Design review of the part built by this model. Coordinates are the model's own, in mm. A direction names the side the tool comes from. Give positions to 0.01 mm unless a question says otherwise; leave off trailing zeros. Write each loop counter-clockwise with the first axis right and the second up, starting at its lowest first coordinate (ties: lowest second). Pieces come first, ordered by that corner, then holes.
```python
from build123d import *

# Parameters (mm, degrees)
SALIENTE_EXTRUIR1_DEPTH = 1.25
CHAFL_N1_SIZE           = 1.5
CHAFL_N2_SIZE           = 6
CHAFL_N2_SIZE2          = 3
REDONDEO1_R             = 2
REDONDEO2_R             = 10
REDONDEO2_2_R           = 5
REDONDEO3_R             = 0.8
CROQUIS6_R              = 1.2
CROQUIS6_R_2            = 1.7
CORTAR_EXTRUIR1_DEPTH   = 3.5


with BuildPart() as part:
    # Croquis5 → Saliente-Extruir1 (new body, symmetric)
    with BuildSketch(Plane.XY):
        Polygon((-33.3960961, -67.058199354), (-49.468312924, -54.332876319), (-49.042492677, -42.832876319), (-75.361903804, -2.692016862), (-89.503725327, 7.973817187), (-89.503725327, 13.973817187), (-83.503725327, 13.973817187), (-83.503725327, 33.973817187), (-108.003725327, 33.973817187), (-113.503725327, 33.973817187), (-113.503725327, 40.973817187), (-83.503725327, 40.973817187), (-76.07625416, 40.973817187), (-46.8531225, 19.949817187), (-27.852472036, -53.120185426), (-23.157930014, -60.798809991), align=None)
        Polygon((-51.475681089, 9.911759166), (-40.150790084, -33.639898021), (-44.730652374, -36.642805286), (-66.937655512, -2.77395512), align=None, mode=Mode.SUBTRACT)
        Polygon((-72.503725327, 4.947596176), (-56.268652183, 18.267596176), (-72.503725327, 29.947596176), align=None, mode=Mode.SUBTRACT)
    extrude(amount=SALIENTE_EXTRUIR1_DEPTH, both=True)

    # Chafl_n1
    chafl_n1_edges = [part.edges().sort_by_distance(p)[0] for p in [
        (-113.503725327, 33.973817187, 0),
        (-89.503725327, 13.973817187, 0),
    ]]
    chamfer(chafl_n1_edges, length=CHAFL_N1_SIZE)

    # Chafl_n2
    chafl_n2_edges = [part.edges().sort_by_distance(p)[0] for p in [
        (-113.503725327, 40.973817187, 0),
    ]]
    chafl_n2_side = [part.faces().sort_by_distance(p)[0] for p in [
        (-94.789989743, 40.973817187, 0),
    ]]
    chamfer(chafl_n2_edges, length=CHAFL_N2_SIZE, length2=CHAFL_N2_SIZE2, reference=chafl_n2_side[0])

    # Redondeo1
    redondeo1_edges = [part.edges().sort_by_distance(p)[0] for p in [
        (-23.157930014, -60.798809991, 0),
        (-33.3960961, -67.058199354, 0),
        (-51.475681089, 9.911759166, 0),
        (-66.937655512, -2.77395512, 0),
        (-44.730652374, -36.642805286, 0),
        (-40.150790084, -33.639898021, 0),
        (-56.268652183, 18.267596176, 0),
        (-72.503725327, 29.947596176, 0),
        (-72.503725327, 4.947596176, 0),
    ]]
    fillet(redondeo1_edges, radius=REDONDEO1_R)

    # Redondeo2
    redondeo2_edges = [part.edges().sort_by_distance(p)[0] for p in [
        (-76.07625416, 40.973817187, 0),
        (-46.8531225, 19.949817187, 0),
        (-75.361903804, -2.692016862, 0),
        (-27.852472036, -53.120185426, 0),
        (-49.042492677, -42.832876319, 0),
    ]]
    fillet(redondeo2_edges, radius=REDONDEO2_R)

    # Redondeo2 2
    redondeo2_2_edges = [part.edges().sort_by_distance(p)[0] for p in [
        (-49.468312924, -54.332876319, 0),
    ]]
    fillet(redondeo2_2_edges, radius=REDONDEO2_2_R)

    # Redondeo3
    redondeo3_edges = [part.edges().sort_by_distance(p)[0] for p in [
        (-83.503725327, 13.973817187, 0),
        (-83.503725327, 33.973817187, 0),
    ]]
    fillet(redondeo3_edges, radius=REDONDEO3_R)

    # Croquis6 → Cortar-Extruir1 (cut, through all)
    with BuildSketch(Plane.XY.offset(1.25)):
        with Locations((-80.003725327, 31.973817187)):
            Circle(CROQUIS6_R)
        with Locations((-80.003725327, 15.973817187)):
            Circle(CROQUIS6_R)
        with Locations((-85.503725327, 37.473817187)):
            Circle(CROQUIS6_R)
        with Locations((-93.503725327, 37.473817187)):
            Circle(CROQUIS6_R)
        with Locations((-101.503725327, 37.473817187)):
            Circle(CROQUIS6_R)
        with Locations((-109.503725327, 37.473817187)):
            Circle(CROQUIS6_R)
        with Locations((-85.503725327, 10.473817187)):
            Circle(CROQUIS6_R)
        with Locations((-51.75750024, 15.82464715)):
            Circle(CROQUIS6_R_2)
        with Locations((-36.753725327, -37.919792915)):
            Circle(CROQUIS6_R_2)
        with Locations((-44.377518673, -51.986696449)):
            Circle(CROQUIS6_R_2)
        Polygon((-39.612609009, -53.277564811), (-33.640345459, -49.626254349), (-38.856503262, -41.094449277), (-44.828766812, -44.745759739), align=None)
    extrude(amount=-CORTAR_EXTRUIR1_DEPTH, mode=Mode.SUBTRACT)


solid = part.part
```
(1) To check wall thickness, follow L1, parallel to Y at x = -93.5, z = 0; L2, parallel to Y at x = -59, z = -1; L3, parallel to Y at x = -59.5, z = 0.35. State the ranges of each line that lie inside material, in increasing order.
Resolved:
L1: y = 33.97 to 36.27, 38.67 to 40.97
L2: y = -27.65 to -14.88, 3.74 to 16.03, 20.23 to 28.69
L3: y = -26.88 to -14.12, 3.33 to 15.62, 20.59 to 29.05
(2) Clearance check with flat-ended pins moving along their axes: P1, Ø2, axis at x = -101.5, y = 37.47, coming from the +Z side; P2, Ø6, axis at x = -35.5, y = -21, coming from the +Z side; P3, Ø1.5, axis at y = -28, z = -0.5, coming from the +X side; P4, Ø1.5, axis at y = -39, z = -1, coming from the -X side. State where each tip first meets the part, or that it passes through.
Resolved:
P1: passes through
P2: stops at z = 1.25
P3: stops at x = -34.19
P4: stops at x = -52.05
(3) Consider section D-D, the plane z = -0.8. Give the number of separate pieces and of enclosed holes in the cut face, then the cut area to 3 significant figures.
Resolved:
separate pieces: 1
enclosed holes: 13
area: 2,220 mm2
(4) Mouldability with a two-part tool opening along Y and no side actions: class faces 1 (the face through (-37.21, -17.14, 0.02)), 2 (the face through (-40.895, -61.121, 0.018)), 3 (the face through (-51.979, 8.275, -0.018)) as pulls with the +Y half, pulls with the -Y half, needs draft (parallel to the pull), parting line crosses it, or undercut.
Resolved:
face 1: pulls with the +Y half
face 2: pulls with the -Y half
face 3: undercut
(5) Consider section A-A, the plane y = 2. Give the boundary of the cut face in (x, z), then the cut area to 3 significant figures.
Resolved:
outline: (-81.58, -1.25) - (-61.12, -1.25) - (-61.12, 1.25) - (-81.58, 1.25) - close; (-49.42, -1.25) - (-42.19, -1.25) - (-42.19, 1.25) - (-49.42, 1.25) - close
area: 69.2 mm2
(6) Consider section C-C, the plane y = -18. Give the boundary of the cut face in (x, z).
Resolved:
outline: (-65.32, -1.25) - (-56.95, -1.25) - (-56.95, 1.25) - (-65.32, 1.25) - close; (-44.22, -1.25) - (-36.98, -1.25) - (-36.98, 1.25) - (-44.22, 1.25) - close
(7) Tool access review of faces 4 (the face through (-49.27, -48.95, 0.02)), 5 (the face through (-72.504, 18, 0)), 6 (the face through (-113.504, 37, 0)): name each direction out of +Z, -Z, +X, -X, +Y, -Y from which nothing blocks a thin tool from reaching the whole face with its end or side.
Resolved:
face 4: +Z, -Z, -X
face 5: +Z, -Z
face 6: +Z, -Z, -X, +Y, -Y
(8) Consider section B-B, the plane x = -62. Give the boundary of the cut face in (y, z).
Resolved:
outline: (-23.07, -1.25) - (-10.3, -1.25) - (-10.3, 1.25) - (-23.07, 1.25) - close; (1.28, -1.25) - (13.57, -1.25) - (13.57, 1.25) - (1.28, 1.25) - close; (22.39, -1.25) - (30.85, -1.25) - (30.85, 1.25) - (22.39, 1.25) - close
